Check sheet for the drawn part. Datum: minimum x, y, z corner. Units: mm. Give positions to 0.01 mm unless a question says otherwise; leave off trailing zeros. Loops run counter-clockwise (first coordinate to the right, second up) from the corner with the lowest first, then second, coordinate; pieces in that order, holes last. Notation, with made-up numbers: (89, 14.5) - (109, 14.5) arc R15 cw to (109, 33.5) - close; hole circle Ø10 at (69, -7.5). An arc over 180 degrees is marked (long way). One line per item, written item: value. Start each with the question number.
1. Gauge pin test, flat ends, axial feed: pin 1 (1 mm diameter, centred on y = 28, z = 1, fed in from -X); pin 2 (1.5 mm diameter, centred on x = 7.5, z = 1, fed in from -Y); pin 3 (2.5 mm diameter, centred on x = 25, y = 40, fed in from -Z); pin 4 (0.9 mm diameter, centred on y = 61, z = 1, fed in from +X). Record the tip position at first contact, or that the pin passes through.
2. Sectioned sample at A-A (y = 40). Record the cut outline in (x, z).
3. Scan lines: L1, parallel to Y at x = 25, z = 1.5; L2, parallel to Y at x = 45, z = 2.8; L3, parallel to Y at x = 26, z = 0.9. Record each from-to range of solid material in increasing order. Write a range as [from, to].
4. Sectioned sample at D-D (x = 32.5). Record the cut outline in (y, z).
5. Sectioned sample at C-C (y = 55). Record the cut outline in (x, z), plus the area to 3 significant figures.
6. Sectioned sample at B-B (z = 2.5). Count the separate pieces of the cut face and the enclosed holes in it, plus the area to 3 significant figures.
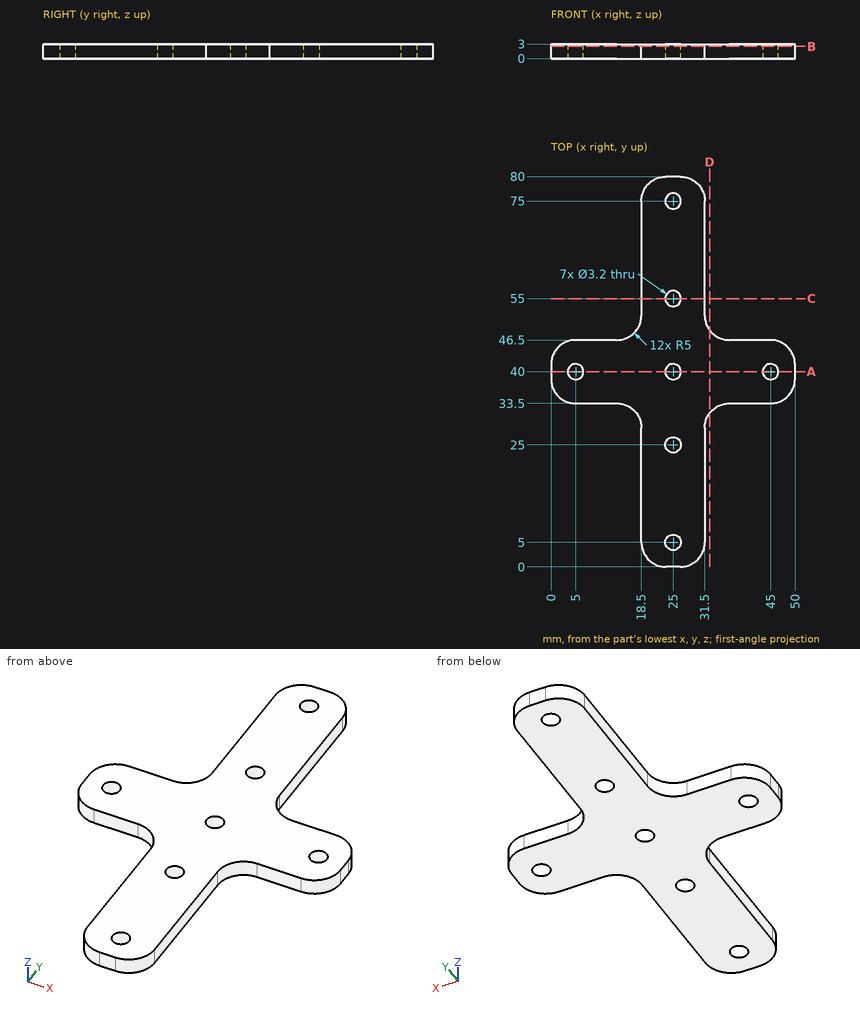
Results are:
1. pin 1: stops at x = 18.5
1. pin 2: stops at y = 33.5
1. pin 3: passes through
1. pin 4: stops at x = 31.5
2. outline: (0, 0) - (3.4, 0) - (3.4, 3) - (0, 3) - close; (6.6, 0) - (23.4, 0) - (23.4, 3) - (6.6, 3) - close; (26.6, 0) - (43.4, 0) - (43.4, 3) - (26.6, 3) - close; (46.6, 0) - (50, 0) - (50, 3) - (46.6, 3) - close
3. L1: y = [0, 3.4], [6.6, 23.4], [26.6, 38.4], [41.6, 53.4], [56.6, 73.4], [76.6, 80]
3. L2: y = [33.5, 38.4], [41.6, 46.5]
3. L3: y = [0, 3.75], [6.25, 23.75], [26.25, 38.75], [41.25, 53.75], [56.25, 73.75], [76.25, 80]
4. outline: (31.5, 0) - (48.5, 0) - (48.5, 3) - (31.5, 3) - close
5. outline: (18.5, 0) - (23.4, 0) - (23.4, 3) - (18.5, 3) - close; (26.6, 0) - (31.5, 0) - (31.5, 3) - (26.6, 3) - close
5. area: 29.4 mm^2
6. separate pieces: 1
6. enclosed holes: 7
6. area: 1,440 mm^2
